Build history of the part. All positions in model axes, mm. Face numbers are marked on the shaded views. Give positions to 0.01 mm unless a question says otherwise; leave off trailing zeros. Order: outer loops, then holes, each group sorted by start corner. A loop starts at its lowest first (then second) coordinate and runs counter-clockwise, first axis right, second up. Notation, with made-up numbers: (-30.75, 17) - (-1.75, 17) arc R22 cw to (-1.75, 55) - close; hole circle Ø10 at (52.5, -24). An arc over 180 degrees is marked (long way). Write each question's results on one line, items separated by ' | '. Start each with the question number.
from build123d import *

# Parameters (mm, degrees)
SKETCH1_R           = 1.825
BOSS_EXTRUDE1_DEPTH = 1.98
SKETCH2_R           = 0.945
BOSS_EXTRUDE2_DEPTH = 12
CUT_EXTRUDE1_DEPTH  = 1
CHAMFER1_SIZE       = 0.2


with BuildPart() as part:
    # Sketch1 → Boss-Extrude1 (new body)
    with BuildSketch(Plane(origin=(0, 0, 0), x_dir=(1, 0, 0), z_dir=(0, 1, 0))):
        Circle(SKETCH1_R)
    extrude(amount=BOSS_EXTRUDE1_DEPTH)

    # Sketch2 → Boss-Extrude2 (add)
    with BuildSketch(Plane(origin=(0, 1.98, 0), x_dir=(1, 0, 0), z_dir=(0, 1, 0))):
        Circle(SKETCH2_R)
    extrude(amount=BOSS_EXTRUDE2_DEPTH)

    # Sketch3 → Cut-Extrude1 (cut)
    with BuildSketch(Plane.XZ):
        Polygon((0.458993464, -0.795), (0.917986928, 0), (0.458993464, 0.795), (-0.458993464, 0.795), (-0.917986928, 0), (-0.458993464, -0.795), align=None)
    extrude(amount=-CUT_EXTRUDE1_DEPTH, mode=Mode.SUBTRACT)

    # Chamfer1
    chamfer1_edges = [part.edges().sort_by_distance(p)[0] for p in [
        (-0.945, 13.98, 0),
    ]]
    chamfer(chamfer1_edges, length=CHAMFER1_SIZE)


solid = part.part
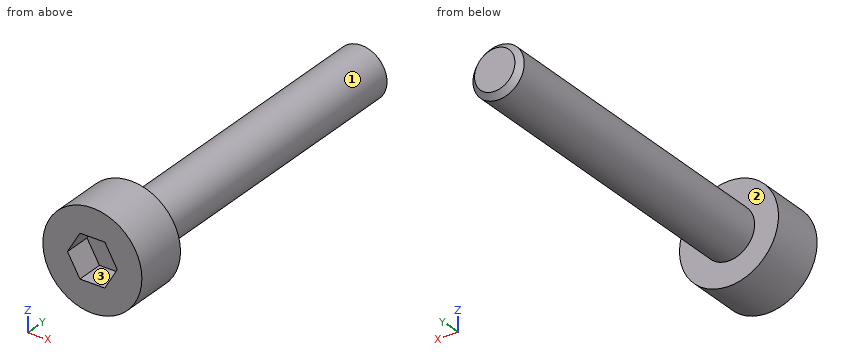
Item 1: Cut at C-C, the plane x = -1.1. List the corners of the cut face in (y, z), then the cut area to 3 significant figures.
Item 2: Probe line 1 along Y through (x, z) = (1.5, -0.55); line 2 along Z through (x, y) = (0, 10) (3 decimals); line 3 along Y through (x, z) = (-0.3, 0.65). List the from-to ranges inside material, lowest first. Write a range as from..to.
Item 3: Two-plate mould, pull along Z, no slides. Class the marked faces 1, 2 and 3: +Z half, -Z half, draft (parallel to the pull), parting line (faces both ways), or undercut.
Item 4: Flat gauge pins, fed straight in: pin 1 Ø1 at (x, z) = (0.5, -1) entering from -Y; pin 2 Ø0.5 at (x, z) = (0, 0.5) entering from -Y. Where does each tip first touch, or does it go through?
Item 5: Cut at A-A, the plane x = 0. List the corners of the cut face in (y, z) (3 decimals), then the cut area to 3 significant figures.
Item 6: Cut at B-B, the plane y = 2.5. List the corners of the cut face in (x, z) (3 decimals).
Values found:
1) outline: (0, -1.46) - (1.98, -1.46) - (1.98, 1.46) - (0, 1.46) - close | area: 5.77 mm2
2) line 1: y = 0..1.98 | line 2: z = -0.945..0.945 | line 3: y = 1..13.98
3) face 1: parting line | face 2: draft | face 3: undercut
4) pin 1: stops at y = 0 | pin 2: stops at y = 1
5) outline: (0, -1.825) - (1.98, -1.825) - (1.98, -0.945) - (13.78, -0.945) - (13.98, -0.745) - (13.98, 0.745) - (13.78, 0.945) - (1.98, 0.945) - (1.98, 1.825) - (0, 1.825) - (0, 0.795) - (1, 0.795) - (1, -0.795) - (0, -0.795) - close | area: 28.3 mm2
6) outline: circle Ø1.89 at (0, 0)
